Can you work these out from the model? Positions are in its coordinate system, mm. A direction names the side the tool comes from. Round coordinates to 2 decimals unless told otherwise and drop trailing zeros. Write each loop counter-clockwise with the first axis right and the second up, starting at its lowest first coordinate (ties: lowest second). Pieces come first, ordered by that corner, then holes.
Q1. If we section it at B-B (z = -14.75): Please give me the cut outline in (x, y).
Q2. If we section it at C-C (y = -10): Please give me the cut outline in (x, z).
Q3. If we section it at D-D (x = 0): Give the number of separate pieces and of enclosed holes in the cut face, plus the area to 3 significant figures.
Q4. If we section it at A-A (y = 0): Please give me the cut outline in (x, z).
Q5. Please list where these lines run through material, in increasing order: line 1 along Y through (x, z) = (0, 4.9); line 2 along Y through (x, z) = (0, 1); line 3 along Y through (x, z) = (-11.5, 1).
Q6. For faces 1 (the flat face through (-36, 18, 4.5)), 2 (the cylindrical face through (18.56, -19.45, 3.3)), which set-ups out of +Z, -Z, +X, -X, +Y, -Y let a thin tool reach every point of the face, with its end or its side?
Q7. I'm going to push flat-ended pins straight in: pin 1 Ø6 at (x, y) = (-36.5, 18.5) entering from -Z; pin 2 Ø5.5 at (x, y) = (0, -40) entering from -Z; pin 3 Ø10 at (y, z) = (7, -8) entering from +X; pin 4 Ø10 at (x, y) = (-21, -0.5) entering from +Z. Where does each tip first touch, or does it pass through?
from build123d import *

# Parameters (mm, degrees)
SKETCH_1_R               = 45
EXTRUDE_1_DEPTH          = 6
SKETCH_2_R               = 34.65
SKETCH_2_R_2             = 2
CUT_EXTRUDE_1_DEPTH      = 64.921827258
EXTRUDE_START            = -3.5
SKETCH_4_R               = 34.65
EXTRUDE_3_DEPTH          = 3.5
SKETCH_5_R               = 15
EXTRUDE_4_DEPTH          = 17
SKETCH_6_R               = 3.75
CUT_EXTRUDE_2_DEPTH      = 4
PATTERN_CIRCULAR_1_COUNT = 6
CUT_EXTRUDE_4_DEPTH      = 66.871086221
CUT_EXTRUDE_5_DEPTH      = 2.5
EXTRUDE_6_DEPTH          = 3
SKETCH_13_R              = 2.1
CUT_EXTRUDE_6_DEPTH      = 5
SKETCH_14_R              = 3.75
CUT_EXTRUDE_7_DEPTH      = 1
HOLE_WIZARD_M4_1_D       = 3.3
FILLET_1_R               = 2
CUT_EXTRUDE_8_DEPTH      = 10
FILLET_2_R               = 2
SKETCH_21_R              = 6
CUT_EXTRUDE_9_DEPTH      = 68


with BuildPart() as part:
    # 草图1 → 凸台-拉伸1 (new body)
    with BuildSketch(Plane.XY):
        Circle(SKETCH_1_R)
    extrude(amount=EXTRUDE_1_DEPTH)

    # 草图2 → 切除-拉伸1 (cut, through all)
    with BuildSketch(Plane.XY.offset(6)):
        Circle(SKETCH_2_R)
        with Locations((0, 40)):
            Circle(SKETCH_2_R_2)
        with Locations((34.641016151, 20)):
            Circle(SKETCH_2_R_2)
        with Locations((34.641016151, -20)):
            Circle(SKETCH_2_R_2)
        with Locations((0, -40)):
            Circle(SKETCH_2_R_2)
        with Locations((-34.641016151, -20)):
            Circle(SKETCH_2_R_2)
        with Locations((-34.641016151, 20)):
            Circle(SKETCH_2_R_2)
    extrude(amount=-CUT_EXTRUDE_1_DEPTH, mode=Mode.SUBTRACT)

    # 草图4 → 凸台-拉伸3 (add)
    with BuildSketch(Plane(origin=(0, 0, 0), x_dir=(-1, 0, 0), z_dir=(0, 0, -1)).offset(EXTRUDE_START)):
        with Locations(Location((0, 0, 0), (0, 0, 180))):
            Circle(SKETCH_4_R)
    extrude(amount=EXTRUDE_3_DEPTH)

    # 草图5 → 凸台-拉伸4 (add)
    with BuildSketch(Plane(origin=(0, 0, 0), x_dir=(-1, 0, 0), z_dir=(0, 0, -1))):
        with Locations(Location((0, 0, 0), (0, 0, 180))):
            Circle(SKETCH_5_R)
    extrude(amount=EXTRUDE_4_DEPTH)

    # 草图6 → 切除-拉伸2 (cut)
    with BuildSketch(Plane(origin=(0, 0, 0), x_dir=(-1, 0, 0), z_dir=(0, 0, -1))):
        with Locations((0, 40)):
            Circle(SKETCH_6_R)
    cut_extrude_2 = extrude(amount=-CUT_EXTRUDE_2_DEPTH, mode=Mode.SUBTRACT)

    # 阵列(圆周)1: 切除-拉伸2 ×6 about axis
    pattern_circular_1_axis = Axis((0, 0, 0), (0, 0, 1))
    for i in range(1, PATTERN_CIRCULAR_1_COUNT):
        add(cut_extrude_2.rotate(pattern_circular_1_axis, i * 360 / PATTERN_CIRCULAR_1_COUNT), mode=Mode.SUBTRACT)

    # 草图9 → 切除-拉伸4 (cut, through all)
    with BuildSketch(Plane(origin=(0, 0, 0), x_dir=(-1, 0, 0), z_dir=(0, 0, -1))):
        Polygon((24.526279442, -20.480762114), (42.026279442, -50.791651246), (22.973720558, -61.791651246), (5.473720558, -31.480762114), align=None)
    extrude(amount=-CUT_EXTRUDE_4_DEPTH, mode=Mode.SUBTRACT)

    # 草图11 → 切除-拉伸5 (cut)
    with BuildSketch(Plane.XY.offset(6)):
        with BuildLine():
            Line((-31.343703671, -32.288887255), (-25.955084176, -22.955524508))
            ThreePointArc((-25.955084176, -22.955524508), (17.325, 30.007780241), (-6.902525293, -33.955524508))
            Line((-6.902525293, -33.955524508), (-12.291144788, -43.288887255))
            ThreePointArc((-12.291144788, -43.288887255), (22.5, 38.97114317), (-31.343703671, -32.288887255))
        make_face()
    extrude(amount=-CUT_EXTRUDE_5_DEPTH, mode=Mode.SUBTRACT)

    # 草图12 → 凸台-拉伸6 (add)
    with BuildSketch(Plane.XY.offset(3.5)):
        with BuildLine():
            Line((-5.473720558, -31.480762114), (-12.291144788, -43.288887255))
            ThreePointArc((-12.291144788, -43.288887255), (22.5, 38.97114317), (-31.343703671, -32.288887255))
            Line((-31.343703671, -32.288887255), (-24.526279442, -20.480762114))
            Line((-24.526279442, -20.480762114), (-5.473720558, -31.480762114))
        make_face()
    extrude(amount=EXTRUDE_6_DEPTH)

    # 草图13 → 切除-拉伸6 (cut)
    with BuildSketch(Plane.XY.offset(6.5)):
        with Locations((0, 40)):
            Circle(SKETCH_13_R)
        with Locations((34.641016151, 20)):
            Circle(SKETCH_13_R)
        with Locations((34.641016151, -20)):
            Circle(SKETCH_13_R)
        with Locations((0, -40)):
            Circle(SKETCH_13_R)
        with Locations((-34.641016151, -20)):
            Circle(SKETCH_13_R)
        with Locations((-34.641016151, 20)):
            Circle(SKETCH_13_R)
    extrude(amount=-CUT_EXTRUDE_6_DEPTH, mode=Mode.SUBTRACT)

    # 草图14 → 切除-拉伸7 (cut)
    with BuildSketch(Plane(origin=(0, 0, 3.5), x_dir=(-1, 0, 0), z_dir=(0, 0, -1))):
        with Locations((0, 40)):
            Circle(SKETCH_14_R)
        with Locations((-34.641016151, 20)):
            Circle(SKETCH_14_R)
        with Locations((34.641016151, 20)):
            Circle(SKETCH_14_R)
        with Locations((34.641016151, -20)):
            Circle(SKETCH_14_R)
        with Locations((0, -40)):
            Circle(SKETCH_14_R)
        with Locations((-34.641016151, -20)):
            Circle(SKETCH_14_R)
    extrude(amount=-CUT_EXTRUDE_7_DEPTH, mode=Mode.SUBTRACT)

    # M4 螺纹孔1 (through all)
    with Locations(Plane(origin=(0, 10, -17), x_dir=(-1, 0, 0), z_dir=(0, 0, -1))):
        with Locations((0, 0), (10, -10), (0, -20), (-10, -10)):
            Hole(HOLE_WIZARD_M4_1_D / 2)

    # 圆角1
    fillet_1_edges = [part.edges().sort_by_distance(p)[0] for p in [
        (-12.291144788, -43.288887255, 3.25),
        (-5.473720558, -31.480762114, 3.25),
        (-31.343703671, -32.288887255, 3.25),
        (-24.526279442, -20.480762114, 3.25),
    ]]
    fillet(fillet_1_edges, radius=FILLET_1_R)

    # 草图20 → 切除-拉伸8 (cut)
    with BuildSketch(Plane(origin=(0, 0, 0), x_dir=(-1, 0, 0), z_dir=(0, 0, -1))):
        with BuildLine():
            Line((-4.529333289, 16.90370196), (-7.11752374, 26.562960223))
            ThreePointArc((-7.11752374, 26.562960223), (-13.75, 23.815698604), (-19.445436483, 19.445436483))
            Line((-19.445436483, 19.445436483), (-12.374368671, 12.374368671))
            ThreePointArc((-12.374368671, 12.374368671), (-8.75, 15.155444566), (-4.529333289, 16.90370196))
        make_face()
        with BuildLine():
            Line((12.374368671, 12.374368671), (19.445436483, 19.445436483))
            ThreePointArc((19.445436483, 19.445436483), (13.75, 23.815698604), (7.11752374, 26.562960223))
            Line((7.11752374, 26.562960223), (4.529333289, 16.90370196))
            ThreePointArc((4.529333289, 16.90370196), (8.75, 15.155444566), (12.374368671, 12.374368671))
        make_face()
        with BuildLine():
            Line((16.90370196, -4.529333289), (26.562960223, -7.11752374))
            ThreePointArc((26.562960223, -7.11752374), (27.5, 0), (26.562960223, 7.11752374))
            Line((26.562960223, 7.11752374), (16.90370196, 4.529333289))
            ThreePointArc((16.90370196, 4.529333289), (17.5, 0), (16.90370196, -4.529333289))
        make_face()
        with BuildLine():
            Line((4.529333289, -16.90370196), (7.11752374, -26.562960223))
            ThreePointArc((7.11752374, -26.562960223), (13.75, -23.815698604), (19.445436483, -19.445436483))
            Line((19.445436483, -19.445436483), (12.374368671, -12.374368671))
            ThreePointArc((12.374368671, -12.374368671), (8.75, -15.155444566), (4.529333289, -16.90370196))
        make_face()
        with BuildLine():
            Line((-12.374368671, -12.374368671), (-19.445436483, -19.445436483))
            ThreePointArc((-19.445436483, -19.445436483), (-13.75, -23.815698604), (-7.11752374, -26.562960223))
            Line((-7.11752374, -26.562960223), (-4.529333289, -16.90370196))
            ThreePointArc((-4.529333289, -16.90370196), (-8.75, -15.155444566), (-12.374368671, -12.374368671))
        make_face()
        with BuildLine():
            Line((-16.90370196, 4.529333289), (-26.562960223, 7.11752374))
            ThreePointArc((-26.562960223, 7.11752374), (-27.5, 0), (-26.562960223, -7.11752374))
            Line((-26.562960223, -7.11752374), (-16.90370196, -4.529333289))
            ThreePointArc((-16.90370196, -4.529333289), (-17.5, 0), (-16.90370196, 4.529333289))
        make_face()
    extrude(amount=-CUT_EXTRUDE_8_DEPTH, mode=Mode.SUBTRACT)

    # 圆角2
    fillet_2_edges = [part.edges().sort_by_distance(p)[0] for p in [
        (-12.374368671, 12.374368671, 3.25),
        (-4.529333289, 16.90370196, 3.25),
        (-7.11752374, 26.562960223, 3.25),
        (-19.445436483, 19.445436483, 3.25),
        (-16.90370196, -4.529333289, 3.25),
        (-16.90370196, 4.529333289, 3.25),
        (-26.562960223, 7.11752374, 3.25),
        (-26.562960223, -7.11752374, 3.25),
        (-4.529333289, -16.90370196, 3.25),
        (-12.374368671, -12.374368671, 3.25),
        (-19.445436483, -19.445436483, 3.25),
        (-7.11752374, -26.562960223, 3.25),
        (12.374368671, -12.374368671, 3.25),
        (4.529333289, -16.90370196, 3.25),
        (7.11752374, -26.562960223, 3.25),
        (19.445436483, -19.445436483, 3.25),
        (16.90370196, 4.529333289, 3.25),
        (16.90370196, -4.529333289, 3.25),
        (26.562960223, -7.11752374, 3.25),
        (26.562960223, 7.11752374, 3.25),
        (4.529333289, 16.90370196, 3.25),
        (12.374368671, 12.374368671, 3.25),
        (19.445436483, 19.445436483, 3.25),
        (7.11752374, 26.562960223, 3.25),
    ]]
    fillet(fillet_2_edges, radius=FILLET_2_R)

    # 草图21 → 切除-拉伸9 (cut)
    with BuildSketch(Plane(origin=(0, 0, -17), x_dir=(-1, 0, 0), z_dir=(0, 0, -1))):
        Circle(SKETCH_21_R)
    extrude(amount=-CUT_EXTRUDE_9_DEPTH, mode=Mode.SUBTRACT)


solid = part.part
A:
1. outline: circle Ø30 at (0, 0); hole circle Ø3.3 at (-10, 0); hole circle Ø12 at (0, 0); hole circle Ø3.3 at (0, -10); hole circle Ø3.3 at (0, 10); hole circle Ø3.3 at (10, 0)
2. outline: (-43.87, 0) - (-11.18, 0) - (-11.18, -17) - (-1.65, -17) - (-1.65, 6.5) - (-43.87, 6.5) - close; (1.65, -17) - (11.18, -17) - (11.18, 0) - (43.87, 0) - (43.87, 6.5) - (1.65, 6.5) - close
3. separate pieces: 6
3. enclosed holes: 0
3. area: 574 mm2
4. outline: (-45, 0) - (-27.5, 0) - (-27.5, 6.5) - (-45, 6.5) - close; (-17.5, 0) - (-15, 0) - (-15, -17) - (-11.65, -17) - (-11.65, 6.5) - (-17.5, 6.5) - close; (-8.35, -17) - (-6, -17) - (-6, 6.5) - (-8.35, 6.5) - close; (6, -17) - (8.35, -17) - (8.35, 6.5) - (6, 6.5) - close; (11.65, -17) - (15, -17) - (15, 0) - (17.5, 0) - (17.5, 6.5) - (11.65, 6.5) - close; (27.5, 0) - (45, 0) - (45, 6.5) - (27.5, 6.5) - close
5. line 1: y = -45 to -42.1, -37.9 to -11.65, -8.35 to -6, 6 to 8.35, 11.65 to 37.9, 42.1 to 45
5. line 2: y = -45 to -43.75, -36.25 to -11.65, -8.35 to -6, 6 to 8.35, 11.65 to 36.25, 43.75 to 45
5. line 3: y = -28 to -24.98, -13.3 to -0.69, 0.69 to 13.3, 24.98 to 43.51
6. face 1: -Z
6. face 2: +Z, -Z
7. pin 1: stops at z = 0
7. pin 2: stops at z = 4.5
7. pin 3: stops at x = 14.87
7. pin 4: stops at z = 6.5
